from build123d import *

# Parameters (mm, degrees)
F0_R      = 254
F1_DEPTH  = 25.4
F3_R      = 254
F4_DEPTH  = 50.8
F6_DEPTH  = 127
F8_DEPTH  = 152.4
F9_R      = 127
F10_DEPTH = 127
F11_R     = 21.463
F12_DEPTH = 152.401
F13_R     = 11.1125
F14_DEPTH = 50.801


with BuildPart() as f1:
    # F0 (on Top) → F1 (new body)
    with BuildSketch(Plane.XY):
        Circle(F0_R)
    extrude(amount=F1_DEPTH)



with BuildPart() as f4:
    # F3 (on offset) → F4 (new body)
    with BuildSketch(Plane.XY.offset(152.4)):
        with BuildLine():
            ThreePointArc((-305.1073144143, -153.3185779875), (-304.6298197167, -155.3799861666), (-303.8166886514, -157.3335016483))
            ThreePointArc((-303.8166886514, -157.3335016483), (-241.9280999016, -241.9280999016), (-157.3335016483, -303.8166886514))
            ThreePointArc((-157.3335016483, -303.8166886514), (-155.3799861666, -304.6298197167), (-153.3185779875, -305.1073144143))
            ThreePointArc((-153.3185779875, -305.1073144143), (0, -316.1821353814), (153.3185779875, -305.1073144143))
            ThreePointArc((153.3185779875, -305.1073144143), (155.3799861666, -304.6298197167), (157.3335016483, -303.8166886514))
            ThreePointArc((157.3335016483, -303.8166886514), (241.9280999016, -241.9280999016), (303.8166886514, -157.3335016483))
            ThreePointArc((303.8166886514, -157.3335016483), (304.6298197167, -155.3799861666), (305.1073144143, -153.3185779875))
            ThreePointArc((305.1073144143, -153.3185779875), (316.1821353814, 0), (305.1073144143, 153.3185779875))
            ThreePointArc((305.1073144143, 153.3185779875), (304.6298197167, 155.3799861666), (303.8166886514, 157.3335016483))
            ThreePointArc((303.8166886514, 157.3335016483), (241.9280999016, 241.9280999016), (157.3335016483, 303.8166886514))
            ThreePointArc((157.3335016483, 303.8166886514), (155.3799861666, 304.6298197167), (153.3185779875, 305.1073144143))
            ThreePointArc((153.3185779875, 305.1073144143), (0, 316.1821353814), (-153.3185779875, 305.1073144143))
            ThreePointArc((-153.3185779875, 305.1073144143), (-155.3799861666, 304.6298197167), (-157.3335016483, 303.8166886514))
            ThreePointArc((-157.3335016483, 303.8166886514), (-241.9280999016, 241.9280999016), (-303.8166886514, 157.3335016483))
            ThreePointArc((-303.8166886514, 157.3335016483), (-304.6298197167, 155.3799861666), (-305.1073144143, 153.3185779875))
            ThreePointArc((-305.1073144143, 153.3185779875), (-316.1821353814, 0), (-305.1073144143, -153.3185779875))
        make_face()
        Circle(F3_R, mode=Mode.SUBTRACT)
    extrude(amount=-F4_DEPTH)


with BuildPart() as f1_1:
    add(f1.part)

    add(f4.part)  # F6 merges F4
    # F5 (on Front) → F6 (join, symmetric)
    with BuildSketch(Plane.XZ):
        Polygon((-279.2956233025, 105.3081825376), (-203.2, 0), (-196.8173876795, 17.664473254), (-260.1486742496, 105.3081825376), align=None)
        Polygon((196.8173876795, 17.664473254), (203.2, 0), (279.2956233025, 105.3081825376), (260.1486742496, 105.3081825376), align=None)
    extrude(amount=F6_DEPTH, both=True)

    # F7 (on Right) → F8 (join, symmetric)
    with BuildSketch(Plane.YZ):
        Polygon((165.1, 23.3656521887), (203.2, 23.3656521887), (278.463602066, 101.9842028618), (240.363602066, 101.9842028618), align=None)
        Polygon((-278.463602066, 101.9842028618), (-203.2, 23.3656521887), (-165.1, 23.3656521887), (-240.363602066, 101.9842028618), align=None)
    extrude(amount=F8_DEPTH, both=True)

    # F9 (on face) → F10 (join)
    with BuildSketch(Plane.XY.offset(25.4)):
        Circle(F9_R)
    extrude(amount=F10_DEPTH)

    # F11 (on face) → F12 (cut, through all)
    with BuildSketch(Plane.XY.offset(152.4)):
        Circle(F11_R)
    extrude(amount=-F12_DEPTH, mode=Mode.SUBTRACT)

    # F13 (on face) → F14 (cut, through all)
    with BuildSketch(Plane(origin=(0, 0, 101.6), x_dir=(1, 0, 0), z_dir=(0, 0, -1))):
        with Locations((219.075, 219.075)):
            Circle(F13_R)
        with Locations((219.075, -219.075)):
            Circle(F13_R)
        with Locations((-219.075, -219.075)):
            Circle(F13_R)
        with Locations((-219.075, 219.075)):
            Circle(F13_R)
    extrude(amount=-F14_DEPTH, mode=Mode.SUBTRACT)


solid = f1_1.part
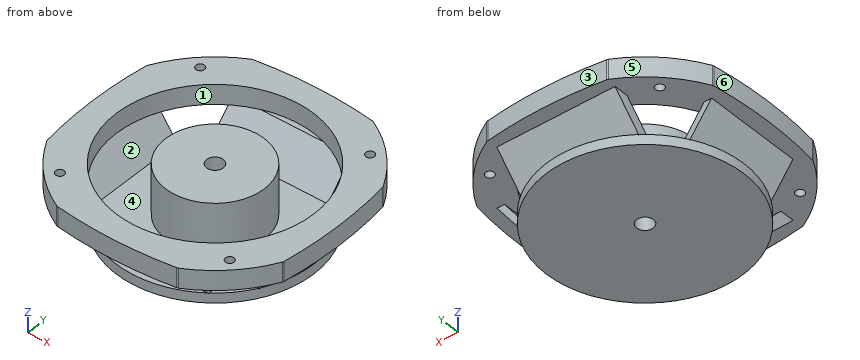
Input: part model. Units: mm. Frame: model coordinates. Face numbers are marked on the shaded views. A direction names the side the tool comes from. Coordinates: 2 decimals unless noted, no trailing zeros. Order: outer loops, then holes, each group sorted by start corner. A loop starts at its lowest first (then second) coordinate and runs counter-clockwise, first axis right, second up.
1. Access query for the marked faces 1, 2 and 3. Directions: +Z, -Z, +X, -X, +Y, -Y. A direction counts if a zero-diameter tool reaches every point of the face in a straight line with its end or side. Return the directions, or none.
Checked values:
face 1: +Z
face 2: +Y, -Y
face 3: +Z, -Z, +Y
2. Cut plane B-B, the plane y = 0. Return loops of the section in (x, z), plus the area to 3 significant figures.
Checked values:
outline: (-316.18, 101.6) - (-276.62, 101.6) - (-221.55, 25.4) - (-254, 25.4) - (-254, 0) - (-21.46, 0) - (-21.46, 152.4) - (-127, 152.4) - (-127, 25.4) - (-202.41, 25.4) - (-257.47, 101.6) - (-254, 101.6) - (-254, 152.4) - (-316.18, 152.4) - close; (21.46, 0) - (254, 0) - (254, 25.4) - (221.55, 25.4) - (276.62, 101.6) - (316.18, 101.6) - (316.18, 152.4) - (254, 152.4) - (254, 101.6) - (257.47, 101.6) - (202.41, 25.4) - (127, 25.4) - (127, 152.4) - (21.46, 152.4) - close
area: 47,900 mm2
3. Ray query, line 1 along Y through (x, z) = (7, 28.5); line 2 along Y through (x, z) = (22, 116); line 3 along Y through (x, z) = (-113.5, 90). Return the intervals inside material, ascending.
Checked values:
line 1: y = -208.12 to -170.02, -126.81 to -20.29, 20.29 to 126.81, 170.02 to 208.12
line 2: y = -315.96 to -253.05, -125.08 to 125.08, 253.05 to 315.96
line 3: y = -266.99 to -228.89, -56.98 to 56.98, 228.89 to 266.99
4. Draft query along Y for the marked faces 4, 5 and 6. Return one class per face: +Y half, -Y half, draft (parallel to the pull), parting line (faces both ways), or undercut.
Checked values:
face 4: undercut
face 5: +Y half
face 6: parting line
5. Contact query for flat-ended pins moving along their axis: P1, Ø10, axis at y = -242, z = 98, coming from the +X side; P2, Ø9.5, axis at x = -233, y = 41, coming from the +Z side; P3, Ø4, axis at y = -128.5, z = 81, coming from the -X side; P4, Ø13.5, axis at x = -219.075, y = -219.075, coming from the +Z side. Output: stop coordinate, or through.
Checked values:
P1: stops at x = 245.28
P2: stops at z = 74.31
P3: stops at x = -262.69
P4: passes through
6. Cut plane A-A, the plane x = 0. Return loops of the section in (y, z), plus the area to 3 significant figures.
Checked values:
outline: (-316.18, 101.6) - (-278.1, 101.6) - (-205.15, 25.4) - (-254, 25.4) - (-254, 0) - (-21.46, 0) - (-21.46, 152.4) - (-127, 152.4) - (-127, 25.4) - (-167.05, 25.4) - (-240.36, 101.98) - (-254, 101.98) - (-254, 152.4) - (-316.18, 152.4) - close; (21.46, 0) - (254, 0) - (254, 25.4) - (205.15, 25.4) - (278.1, 101.6) - (316.18, 101.6) - (316.18, 152.4) - (254, 152.4) - (254, 101.98) - (240.36, 101.98) - (167.05, 25.4) - (127, 25.4) - (127, 152.4) - (21.46, 152.4) - close
area: 50,800 mm2
7. Cut plane D-D, the plane y = -145. Return loops of the section in (x, z).
Checked values:
outline: (-306.28, 101.6) - (-208.54, 101.6) - (-208.54, 152.4) - (-306.28, 152.4) - close; (-208.54, 0) - (208.54, 0) - (208.54, 25.4) - (-208.54, 25.4) - close; (208.54, 101.6) - (306.28, 101.6) - (306.28, 152.4) - (208.54, 152.4) - close
8. Cut plane C-C, the plane z = 123.5. Return loops of the section in (x, y) (1 decimal).
Checked values:
outline: (-305.1, -153.3) arc R12.7 ccw to (-303.8, -157.3) arc R342.1 ccw to (-157.3, -303.8) arc R12.7 ccw to (-153.3, -305.1) arc R1066.8 ccw to (153.3, -305.1) arc R12.7 ccw to (157.3, -303.8) arc R342.1 ccw to (303.8, -157.3) arc R12.7 ccw to (305.1, -153.3) arc R1066.8 ccw to (305.1, 153.3) arc R12.7 ccw to (303.8, 157.3) arc R342.1 ccw to (157.3, 303.8) arc R12.7 ccw to (153.3, 305.1) arc R1066.8 ccw to (-153.3, 305.1) arc R12.7 ccw to (-157.3, 303.8) arc R342.1 ccw to (-303.8, 157.3) arc R12.7 ccw to (-305.1, 153.3) arc R1066.8 ccw to start; circle Ø254 at (0, 0); hole circle Ø508 at (0, 0); hole circle Ø22.2 at (-219.1, -219.1); hole circle Ø22.2 at (-219.1, 219.1); hole circle Ø42.9 at (0, 0); hole circle Ø22.2 at (219.1, -219.1); hole circle Ø22.2 at (219.1, 219.1)
